For this review, use the dimensioned drawing (mm, ordinates from the lowest corner) and the shaded views. Give positions to 0.01 mm unless a question says otherwise; leave off trailing zeros. Loops run counter-clockwise (first coordinate to the right, second up) from the corner with the lowest first, then second, coordinate; pieces in that order, holes last. Notation, with made-up numbers: (-23.5, 28) -> (-13.5, 28) arc R37 cw to (-13.5, 65) -> close; hole circle Ø11 at (79, -12.5). An arc over 180 degrees is marked (long way). Use a Markdown table: item, result. Add a question column.
1. Add section C-C (x = 12.5). State the section outline as (y, z) points.
2. Draft analysis for pull direction Z (two halves, no side actions). For the marked faces 1, 2, 3 and 4, state which applies: pulls with the +Z half, pulls with the -Z half, needs draft (parallel to the pull), parting line crosses it, or undercut.
3. For pin 1 Ø4 at (y, z) = (9, 4) entering from -X; pin 2 Ø6.5 at (x, z) = (15.58, 12.5) entering from -Y, all flat-tipped, find the tip position at first contact; note any pin that passes through.
4. To check wall thickness, follow line 1 (Z direction, x = 19, y = 23) (1 decimal); line 2 (X direction, y = 7.5, z = 11.5); line 3 (X direction, y = 11.5, z = 8.5) (1 decimal). State the ranges of each line that lie inside material, in increasing order.
5. Add section A-A (z = 12.5). State the section outline as (x, y) points.
6. Add section B-B (y = 21). State the section outline as (x, z) points.
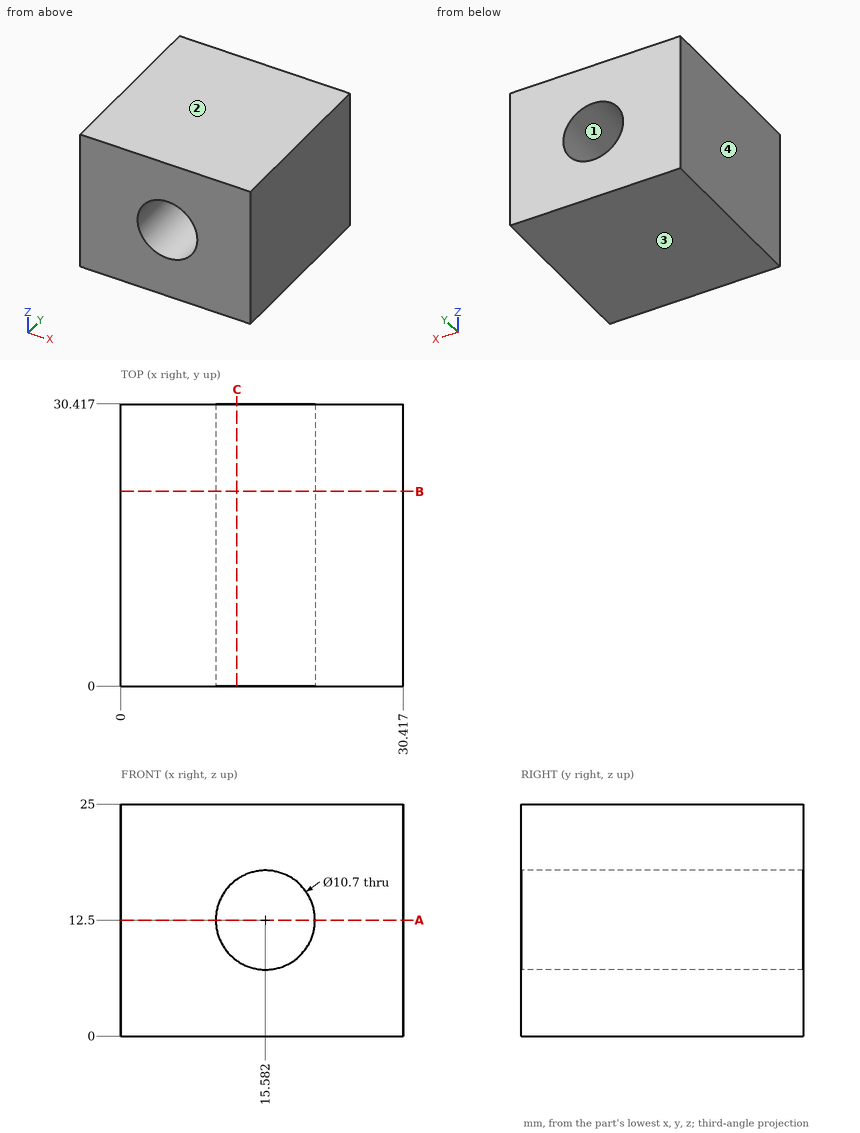
Taken from the geometry:
| question | item | result |
|---|---|---|
| 1 | outline | (0, 0) -> (30.42, 0) -> (30.42, 8.13) -> (0, 8.13) -> close; (0, 16.87) -> (30.42, 16.87) -> (30.42, 25) -> (0, 25) -> close |
| 2 | face 1 | undercut |
| 2 | face 2 | pulls with the +Z half |
| 2 | face 3 | pulls with the -Z half |
| 2 | face 4 | needs draft |
| 3 | pin 1 | stops at x = 0 |
| 3 | pin 2 | passes through |
| 4 | line 1 | z = 0 to 8.4, 16.6 to 25 |
| 4 | line 2 | x = 0 to 10.33, 20.84 to 30.42 |
| 4 | line 3 | x = 0 to 12, 19.1 to 30.4 |
| 5 | outline | (0, 0) -> (10.23, 0) -> (10.23, 30.42) -> (0, 30.42) -> close; (20.93, 0) -> (30.42, 0) -> (30.42, 30.42) -> (20.93, 30.42) -> close |
| 6 | outline | (0, 0) -> (30.42, 0) -> (30.42, 25) -> (0, 25) -> close; hole circle Ø10.7 at (15.58, 12.5) |
